Could you check a few things on this model? Use its own coordinates, in mm. A direction names the side the tool comes from. Round coordinates to 2 decimals unless told otherwise and drop trailing zeros. Loops run counter-clockwise (first coordinate to the right, second up) from the corner with the lowest first, then second, coordinate; pieces in that order, holes last.
from build123d import *

# Parameters (mm, degrees)
F1_W     = 13.8574047014
F1_H     = 58.3990514278
F2_DEPTH = 6.35
F0_W     = 13.97
F0_H     = 30.48
F3_DEPTH = 6.35
F4_R     = 5.08
F6_DEPTH = 14.224


with BuildPart() as f2:
    # F1 (on Top) → F2 (new body)
    with BuildSketch(Plane.XY):
        with Locations((-15.3421224095, -29.1995257139)):
            Rectangle(F1_W, F1_H)
    extrude(amount=F2_DEPTH)

    # F0 (on Front) → F3 (join)
    with BuildSketch(Plane.XZ):
        with Locations((-15.5518442771, 15.24)):
            Rectangle(F0_W, F0_H)
    extrude(amount=F3_DEPTH)

    # F4
    f4_edges = [f2.edges().sort_by_distance(p)[0] for p in [
        (-15.342122, -58.399051, 6.35),
        (-15.551844, -6.35, 30.48),
    ]]
    fillet(f4_edges, radius=F4_R)

    # F5 (on face) → F6 (join)
    with BuildSketch(Plane.YZ.offset(-8.4134200588)):
        Polygon((0, 0), (-58.3990514278, 0), (0, -6.2688249163), align=None)
    extrude(amount=-F6_DEPTH)


solid = f2.part
Item 1: If we section it at C-C, the plane z = 10: Please give me the cut outline in (x, y).
Results list:
outline: (-22.54, -6.35) - (-8.57, -6.35) - (-8.57, 0) - (-22.54, 0) - close
Item 2: If we section it at D-D, the plane y = -16: Please give me the cut outline in (x, z), then the cut area to 3 significant figures.
Results list:
outline: (-22.64, -4.55) - (-8.41, -4.55) - (-8.41, 6.35) - (-22.27, 6.35) - (-22.27, 0) - (-22.64, 0) - close
area: 153 mm2
Item 3: If I drill on line 1 along Y through (x, z) = (-20.5, 17); line 2 along X through (y, z) = (-16.5, 2); line 3 along Z through (x, y) = (-10, -26.5), over which ranges is the centre line in solid material (lowest first)?
Results list:
line 1: y = -6.35 to 0
line 2: x = -22.27 to -8.41
line 3: z = -3.42 to 6.35
Item 4: If we section it at A-A, the plane x = -10.5: Please give me the cut outline in (y, z), then the cut area to 3 significant figures.
Results list:
outline: (-58.4, 0) - (0, -6.27) - (0, 30.48) - (-1.27, 30.48) arc R5.08 ccw to (-6.35, 25.4) - (-6.35, 6.35) - (-53.32, 6.35) arc R5.08 ccw to (-58.4, 1.27) - close
area: 696 mm2
Item 5: For faces 1 (the flat face through (-8.567, -3, 18)), 2 (the flat face through (-22.271, -33, 3)), 3 (the flat face through (-22.537, -3, 15)), which set-ups out of +Z, -Z, +X, -X, +Y, -Y let a thin tool reach every point of the face, with its end or its side?
Results list:
face 1: +Z, +X, +Y, -Y
face 2: +Z, -X, -Y
face 3: +Z, -X, +Y, -Y
Item 6: Will these pins go through, and if not, where does the flat tip stop? pin 1 (5 mm diameter, centred on y = -43, z = 2, fed in from -X); pin 2 (8 mm diameter, centred on y = -8, z = 22, fed in from +X); pin 3 (5 mm diameter, centred on y = -4, z = 16.5, fed in from -X); pin 4 (3 mm diameter, centred on x = -12, y = -19.5, fed in from +Z).
Results list:
pin 1: stops at x = -22.64
pin 2: stops at x = -8.57
pin 3: stops at x = -22.54
pin 4: stops at z = 6.35
Item 7: If we section it at B-B, the plane y = -36.5: Please give me the cut outline in (x, z).
Results list:
outline: (-22.64, -2.35) - (-8.41, -2.35) - (-8.41, 6.35) - (-22.27, 6.35) - (-22.27, 0) - (-22.64, 0) - close
